Source: CAD feature listing. Evaluate the final solid. Frame: model axes, mm. A direction names the side the tool comes from. Round coordinates to 2 decimals unless told otherwise and drop trailing zeros. Loops run counter-clockwise (first coordinate to the right, second up) from the corner with the lowest first, then second, coordinate; pieces in that order, holes last. Notation, with made-up numbers: (89.5, -1) -> (94.5, -1) arc R27 ccw to (94.5, 29) -> close; hole circle Ø9 at (8.5, -2.75). An arc over 180 degrees is marked (long way). Write item = value, one per line.
Autodesk Inventor part; units mm, degrees
ref_plane "YZ Plane" through (0, 0, 0) normal (1, 0, 0) x (0, 1, 0)
ref_plane "XZ Plane" through (0, 0, 0) normal (0, 1, 0) x (-1, 0, 0)
ref_plane "XY Plane" through (0, 0, 0) normal (0, 0, 1) x (1, 0, 0)
sketch "Boceto1" plane through (0, 0, 0) normal (0, 0, 1) x (1, 0, 0)
  line L0 (-24.1261, 0) -> (26.0802, 0) construction
  line L1 (0, 10.125) -> (-30, 10.125)
  line L2 (-30, 10.125) -> (-30, 15)
  line L3 (-30, 15) -> (-15, 15)
  line L4 (-15, 15) -> (-15, 31)
  line L5 (0, 31) -> (0, 10.125)
  line L6 (-15, 31) -> (-13, 31)
  line L7 (-13, 31) -> (-10, 27.5)
  line L8 (-10, 27.5) -> (-5, 27.5)
  line L9 (-2, 31) -> (0, 31)
  line L10 (-2, 31) -> (-5, 27.5)
  line L11 (-7.5, 27.5) -> (-7.5, 0) construction
  point P0 (0, 0)
  point P1 (0, 20.5625)
  dimension "d0" = 27.5
  dimension "d1" = 31
  dimension "d2" = 10.125
  dimension "d3" = 15
  dimension "d4" = 15
  dimension "d5" = 2
  dimension "d6" = 2
  dimension "d7" = 5
  dimension "d8" = 7.5
  dimension "d9" = 15
revolve "Revolución1" add sketch "Boceto1" angle 360 about axis through (-24.1261, 0, 0) along (1, 0, 0)
sketch "Sketch2" plane through (0, 0, 0) normal (0, 0, 1) x (1, 0, 0)
  circle A0 centre (-25, 0) radius 2.25
  point P0 (0, 0)
  dimension "d11" = 4.5
  dimension "d12" = 25
extrude "Extrusion1" cut sketch "Sketch2" along normal blind 34.25
properties part number "PoleaBrazos"
1. Mould query, pull axis Y, two halves, no side actions, for faces 1 (the face through (-15.21, 5.44, -8.54)), 2 (the face through (-30, 3, -10)), 3 (the face through (-22.395, -3.252, -14.643)). Classes: released by +Y, released by -Y, zero draft, split by the parting line, or undercut.
Evaluation:
face_1 = undercut
face_2 = zero draft
face_3 = split by the parting line
2. Section query C-C (x = -9). Return the cut outline in (y, z) (3 decimals), then the cut area to 3 significant figures.
Evaluation:
outline = circle Ø55 at (0, 0); hole circle Ø20.25 at (0, 0)
area = 2,050 mm²
3. Section query D-D (x = -25). Return the cut outline in (y, z) (3 decimals), then the cut area to 3 significant figures.
Evaluation:
outline = (-2.25, 9.872) -> (-2.25, 14.83) arc R15 ccw (long way) to (2.25, 14.83) -> (2.25, 9.872) arc R10.125 cw (long way) to start
area = 363 mm²
4. Set-up query: faces 4 (the face through (-22.854, -0.676, 12.4)), 5 (the face through (-15, 13.3, 7.3)), 6 (the face through (-0.986, -4.036, 30.736)), 7 (the face through (-7.465, -5.961, -26.846)), 8 (the face through (0, -7.3, 7.3)). Return all of +Z, -Z, +X, -X, +Y, -Y with unobstructed straight access to the full face (end or side cutting, diameter ignored); none if empty.
Evaluation:
face_4 = +Z
face_5 = -X
face_6 = +X, -X
face_7 = none
face_8 = +Z, -Z, +X, +Y, -Y
5. Line query: probe 1 along Z at (x, y) = (-17, 0) (3 decimals); probe 2 along X at (y, z) = (0, 11.7); probe 3 along Z at (x, y) = (-26, 7). Output: solid intervals per line, ascending. Write a range as from..to.
Evaluation:
probe_1 = -15..-10.125, 10.125..15
probe_2 = -30..-27.25, -22.75..0
probe_3 = -13.27..-7.32, 7.32..13.27
6. Section query B-B (z = 0). Return the cut outline in (x, y) (3 decimals), then the cut area to 4 significant figures.
Evaluation:
outline = (-30, -15) -> (-15, -15) -> (-15, -31) -> (-13, -31) -> (-10, -27.5) -> (-5, -27.5) -> (-2, -31) -> (0, -31) -> (0, -10.125) -> (-30, -10.125) -> close; (-30, 10.125) -> (0, 10.125) -> (0, 31) -> (-2, 31) -> (-5, 27.5) -> (-10, 27.5) -> (-13, 31) -> (-15, 31) -> (-15, 15) -> (-30, 15) -> close
area = 716.5 mm²
7. Contact query for flat-ended pins moving along their axis: pin 1 Ø5 at (x, z) = (-20.5, 11) entering from -Y; pin 2 Ø5 at (y, z) = (7, 23) entering from -X; pin 3 Ø12 at (x, y) = (-5.5, 5) entering from -Z. Output: stop coordinate, or through.
Evaluation:
pin_1 = -12.36
pin_2 = -15
pin_3 = -31
8. Section query A-A (y = 0). Return the cut outline in (x, z) (3 decimals), then the cut area to 3 significant figures.
Evaluation:
outline = (-30, -15) -> (-15, -15) -> (-15, -31) -> (-13, -31) -> (-10, -27.5) -> (-5, -27.5) -> (-2, -31) -> (0, -31) -> (0, -10.125) -> (-30, -10.125) -> close; (-30, 10.125) -> (-27.25, 10.125) -> (-27.25, 15) -> (-30, 15) -> close; (-22.75, 10.125) -> (0, 10.125) -> (0, 31) -> (-2, 31) -> (-5, 27.5) -> (-10, 27.5) -> (-13, 31) -> (-15, 31) -> (-15, 15) -> (-22.75, 15) -> close
area = 695 mm²
